Input: part model. Units: mm. Frame: model coordinates. A direction names the side the tool comes from. Coordinates: 2 decimals unless noted, no trailing zeros. Order: outer loops, then holes, each group sorted by start corner. A loop starts at its lowest first (then second) coordinate and runs counter-clockwise, first axis right, second up. Notation, with made-up numbers: (51.5, 74.5) -> (75.5, 74.5) arc R28 ccw to (75.5, 110.5) -> close; hole circle Ø2 at (83, 54). An arc over 180 degrees is marked (long way). One line per question, with ' | ' between items.
```python
from build123d import *

# Parameters (mm, degrees)
SKETCH1_W           = 3.5
SKETCH1_H           = 18.5
SKETCH1_W_2         = 2.8
SKETCH1_H_2         = 2.8
BOSS_EXTRUDE1_DEPTH = 2.5
SKETCH4_W           = 3.5
SKETCH4_H           = 1.549747226
BOSS_EXTRUDE2_DEPTH = 2.5


with BuildPart() as part:
    # Sketch1 → Boss-Extrude1 (new body)
    with BuildSketch(Plane(origin=(0, 0, 0), x_dir=(1, 0, 0), z_dir=(0, 1, 0))):
        with Locations((0, -7.5)):
            Rectangle(SKETCH1_W, SKETCH1_H)
        Rectangle(SKETCH1_W_2, SKETCH1_H_2, mode=Mode.SUBTRACT)
    extrude(amount=BOSS_EXTRUDE1_DEPTH)

    # Sketch4 → Boss-Extrude2 (add)
    with BuildSketch(Plane(origin=(0, 2.5, 0), x_dir=(1, 0, 0), z_dir=(0, 1, 0))):
        with Locations((0, -15.975126387)):
            Rectangle(SKETCH4_W, SKETCH4_H)
    extrude(amount=BOSS_EXTRUDE2_DEPTH)


solid = part.part
```
1. Access query for faces 1 (the face through (0, 2, 16.75)), 2 (the face through (0, 4, 15.2)), 3 (the face through (0, 1, 1.4)). Directions: +Z, -Z, +X, -X, +Y, -Y. A direction counts if a zero-diameter tool reaches every point of the face in a straight line with its end or side. Return the directions, or none.
Recorded:
face 1: +Z, +X, -X, +Y, -Y | face 2: -Z, +X, -X, +Y | face 3: +Y, -Y
2. Cut plane C-C, the plane z = 9.5. Return loops of the section in (x, y), and give its area (3 significant figures).
Recorded:
outline: (-1.75, 0) -> (1.75, 0) -> (1.75, 2.5) -> (-1.75, 2.5) -> close | area: 8.75 mm^2
3. Cut plane D-D, the plane y = 3.9. Return loops of the section in (x, z), and give its area (3 significant figures).
Recorded:
outline: (-1.75, 15.2) -> (1.75, 15.2) -> (1.75, 16.75) -> (-1.75, 16.75) -> close | area: 5.42 mm^2
4. Cut plane B-B, the plane y = 2.05. Return loops of the section in (x, z), and give its area (3 significant figures).
Recorded:
outline: (-1.75, -1.75) -> (1.75, -1.75) -> (1.75, 16.75) -> (-1.75, 16.75) -> close; hole (-1.4, -1.4) -> (1.4, -1.4) -> (1.4, 1.4) -> (-1.4, 1.4) -> close | area: 56.9 mm^2
5. Ray query, line 1 (Z direction, x = 0.2, y = 2.05); line 2 (X direction, y = 0.3, z = 0.25); line 3 (Y direction, x = 0, z = 14.75). Return the intervals inside material, ascending. Write a range as [from, to].
Recorded:
line 1: z = [-1.75, -1.4], [1.4, 16.75] | line 2: x = [-1.75, -1.4], [1.4, 1.75] | line 3: y = [0, 2.5]
6. Cut plane A-A, the plane x = -1.1. Return loops of the section in (y, z), and give its area (3 significant figures).
Recorded:
outline: (0, -1.75) -> (2.5, -1.75) -> (2.5, -1.4) -> (0, -1.4) -> close; (0, 1.4) -> (2.5, 1.4) -> (2.5, 15.2) -> (5, 15.2) -> (5, 16.75) -> (0, 16.75) -> close | area: 43.1 mm^2
7. Pin query (flat end, axial travel): pin 1 Ø1.2 at (x, y) = (1, 4.5) entering from -Z; pin 2 Ø1.5 at (y, z) = (4, 12.5) entering from -X. Return the tip coordinate at first contact, or that it passes through.
Recorded:
pin 1: stops at z = 15.2 | pin 2: passes through
